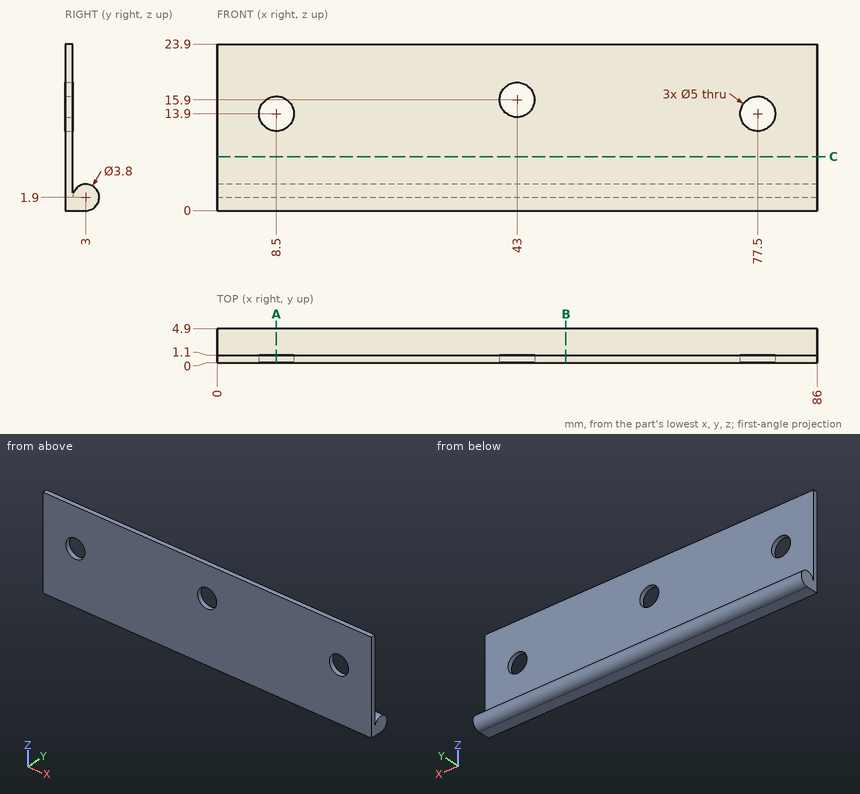
Could you check a few things on this drawing? It's one solid part, dimensions in mm from its lowest x, y, z. Give positions to 0.01 mm unless a question says otherwise; leave off trailing zeros. Order: outer loops, then holes, each group sorted by start corner. A loop starts at its lowest first (then second) coordinate and runs counter-clockwise, first axis right, second up. Notation, with made-up numbers: (-24, -37.75) -> (2, -37.75) arc R19 ccw to (2, -5.75) -> close; hole circle Ø3 at (47, 80.25). An arc over 180 degrees is marked (long way). Answer in a Markdown table with one row per item. Add a question column.
Item 1: I'm going to push flat-ended pins straight in: P1, Ø5, axis at x = 15, z = 15.5, coming from the +Y side; P2, Ø5, axis at x = 39, z = 3, coming from the -Y side. Where does each tip first touch, or does it pass through?
Item 2: Imagine slicing it at A-A (x = 8.5). List the corners of the cut face in (y, z) for me.
Item 3: Imagine slicing it at B-B (x = 50). List the corners of the cut face in (y, z) for me, and give its area (3 significant figures).
Item 4: Imagine slicing it at C-C (z = 7.75). List the corners of the cut face in (x, y) for me.
Item 5: Please list where these lines run through material, in increasing order: probe 1 along X at (y, z) = (0.7, 13.9); probe 2 along Z at (x, y) = (43, 0.65); probe 3 along Z at (x, y) = (8.5, 0.55).
Result:
| question | item | result |
|---|---|---|
| 1 | P1 | y = 1.1 |
| 1 | P2 | y = 0 |
| 2 | outline | (0, 0) -> (3, 0) arc R1.9 ccw (long way) to (1.1, 1.9) -> (1.1, 11.4) -> (0, 11.4) -> close; (0, 16.4) -> (1.1, 16.4) -> (1.1, 23.9) -> (0, 23.9) -> close |
| 3 | outline | (0, 0) -> (3, 0) arc R1.9 ccw (long way) to (1.1, 1.9) -> (1.1, 23.9) -> (0, 23.9) -> close |
| 3 | area | 38.4 mm2 |
| 4 | outline | (0, 0) -> (86, 0) -> (86, 1.1) -> (0, 1.1) -> close |
| 5 | probe 1 | 0 to 6, 11 to 41.5, 44.5 to 75, 80 to 86 |
| 5 | probe 2 | 0 to 13.4, 18.4 to 23.9 |
| 5 | probe 3 | 0 to 11.4, 16.4 to 23.9 |
